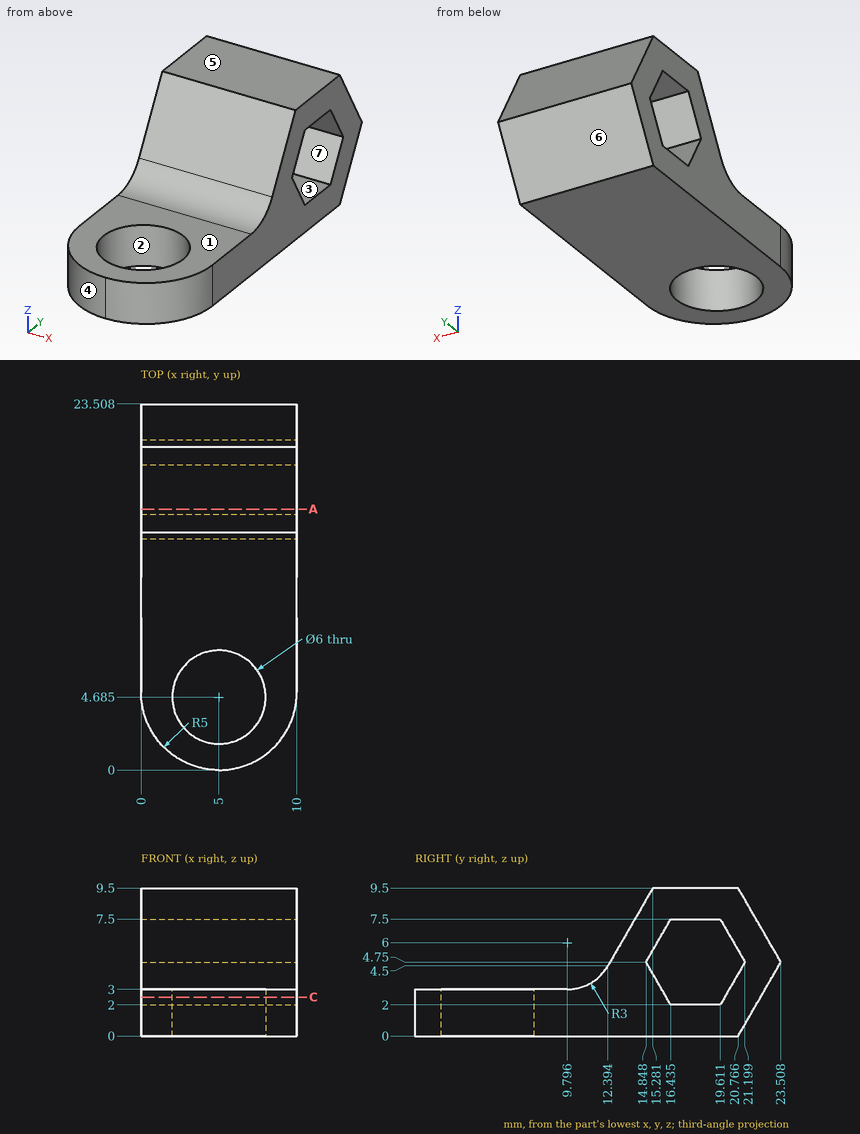
Print and shaded views of the part. All mm, measured from the part's lowest x, y and z. A direction names the side the tool comes from. Coordinates: 2 decimals unless noted, no trailing zeros. Write each loop counter-clockwise with the first axis right and the second up, starting at its lowest first coordinate (ties: lowest second). Pieces come first, ordered by that corner, then holes. Notation, with made-up numbers: (6.5, 42.5) - (21.5, 42.5) arc R15 ccw to (21.5, 55.5) - close; hole circle Ø7 at (1.25, 23.5). An arc over 180 degrees is marked (long way). One line per question, with ' | ' between items. Start each with the question number.
Q1. Pull direction Z, two halves, no side cores. Call the marked faces 4, 5, 6 and 7: pulls with the +Z half, pulls with the -Z half, needs draft (parallel to the pull), parting line crosses it, or undercut.
Q2. Drill centre lines: line 1 (Y direction, x = 5, z = 2.25) (1 decimal); line 2 (Z direction, x = 4.25, y = 18); line 3 (Z direction, x = 8, y = 2.75). Where is each one in solid material? Low to high. Write a range as [from, to].
Q3. Cut at C-C, the plane z = 2.5. Give the number of separate pieces and of enclosed holes in the cut face.
Q4. Pin check, flat tips, straight feed: pin 1 (2 mm diameter, centred on x = 5, z = 7.5, fed in from +Y); pin 2 (5 mm diameter, centred on x = 8.5, z = 2, fed in from -Y); pin 3 (5 mm diameter, centred on x = 5, y = 4.68, fed in from -Z). Stop position of each tip, or through.
Q5. Cut at A-A, the plane y = 16.75. List the corners of the cut face in (x, z).
Q6. 3-axis set-ups, long thin cutter, end or side, ignore diameter. For the marked faces 1, 2 and 3: which of +Z, -Z, +X, -X, +Y, -Y reach the whole face in a straight line?
Answer below:
1) face 4: needs draft | face 5: pulls with the +Z half | face 6: pulls with the -Z half | face 7: undercut
2) line 1: [0, 1.7], [7.7, 16.3], [19.8, 22.1] | line 2: [0, 2], [7.5, 9.5] | line 3: [0, 3]
3) separate pieces: 2 | enclosed holes: 1
4) pin 1: y = 22.5 | pin 2: y = 0.1 | pin 3: through
5) outline: (0, 0) - (10, 0) - (10, 2) - (0, 2) - close; (0, 7.5) - (10, 7.5) - (10, 9.5) - (0, 9.5) - close
6) face 1: +Z, +X, -X, -Y | face 2: +Z, -Z | face 3: +X, -X
